Input: dimensioned drawing with shaded views. Units: mm. Origin: part minimum x, y, z. Round coordinates to 2 decimals unless told otherwise and drop trailing zeros. Write each loop counter-clockwise with the first axis right and the second up, starting at its lowest first coordinate (ties: lowest second). Pieces come first, ordered by that corner, then holes. Notation, with made-up numbers: (89.25, 81) - (147.25, 81) arc R7 cw to (147.25, 90) - close; hole circle Ø5 at (-0.75, 44.5). An arc over 180 degrees is marked (long way). Use one line per item in the form item = value.
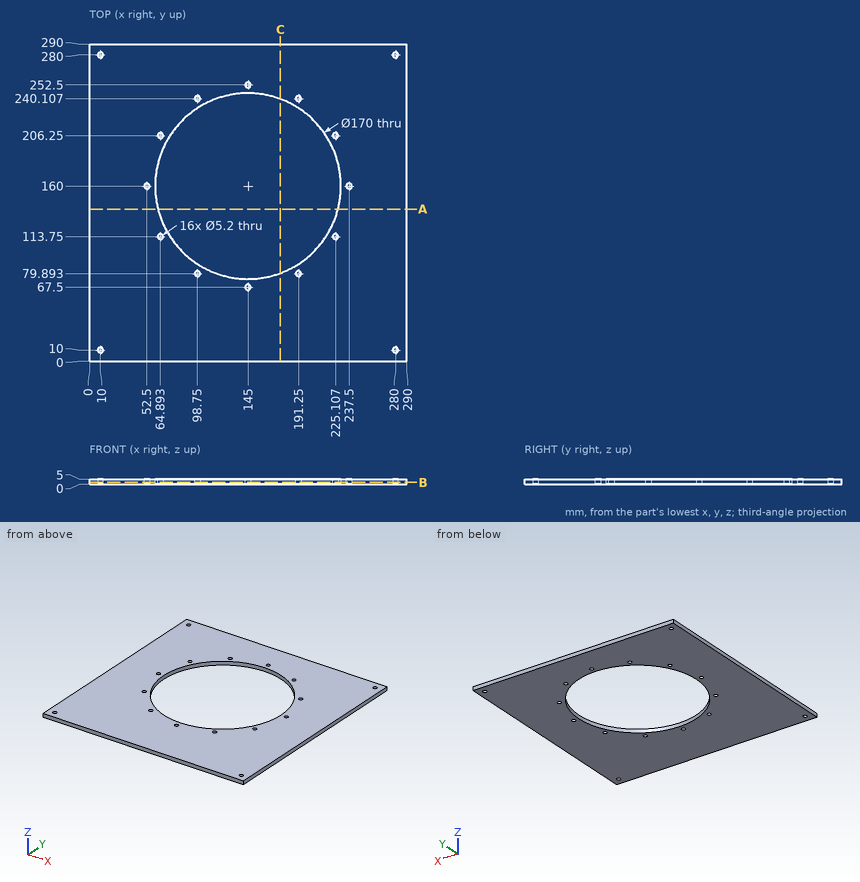
(1) First-contact query: pin 1 Ø4.5 at (x, y) = (145, 252.5) entering from -Z; pin 2 Ø6 at (x, y) = (225.11, 206.25) entering from -Z. Flat tips, straight axial feed; report the tip coordinate or a pass-through.
Derived:
pin_1 = through
pin_2 = 0
(2) Material intervals for L1, parallel to Y at x = 280, z = 2.9; L2, parallel to Y at x = 145, z = 2.3, sorted ascending.
Derived:
L1 = 0 to 7.4, 12.6 to 277.4, 282.6 to 290
L2 = 0 to 64.9, 70.1 to 75, 245 to 249.9, 255.1 to 290
(3) Cut plane B-B on z = 1.95. Count the separate pieces of the cut face and the enclosed holes in it, then the cut area to 3 significant figures.
Derived:
separate_pieces = 1
enclosed_holes = 17
area = 61,100 mm^2
(4) Cut plane A-A on y = 139. Output: boundary loops of the cut face in (x, z) (1 decimal).
Derived:
outline = (0, 0) - (62.6, 0) - (62.6, 5) - (0, 5) - close; (227.4, 0) - (290, 0) - (290, 5) - (227.4, 5) - close
(5) Cut plane C-C on x = 174.5. Output: boundary loops of the cut face in (y, z), then the cut area to 3 significant figures.
Derived:
outline = (0, 0) - (80.28, 0) - (80.28, 5) - (0, 5) - close; (239.72, 0) - (290, 0) - (290, 5) - (239.72, 5) - close
area = 653 mm^2
